from build123d import *

# Parameters (mm, degrees)
SKETCH1_W           = 30
SKETCH1_H           = 30
BOSS_EXTRUDE1_DEPTH = 2
SKETCH2_R           = 1.8
CUT_EXTRUDE1_DEPTH  = 22.307275753
FILLET1_R           = 3
CUT_EXTRUDE2_DEPTH  = 22.307275753


with BuildPart() as part:
    # Sketch1 → Boss-Extrude1 (new body)
    with BuildSketch(Plane.XY):
        Rectangle(SKETCH1_W, SKETCH1_H)
    extrude(amount=BOSS_EXTRUDE1_DEPTH)

    # Sketch2 → Cut-Extrude1 (cut, through all)
    with BuildSketch(Plane.XY.offset(2)):
        with Locations((-12, 12)):
            Circle(SKETCH2_R)
        with Locations((12, 12)):
            Circle(SKETCH2_R)
        with Locations((12, -12)):
            Circle(SKETCH2_R)
        with Locations((-12, -12)):
            Circle(SKETCH2_R)
    extrude(amount=-CUT_EXTRUDE1_DEPTH, mode=Mode.SUBTRACT)

    # Fillet1
    fillet1_edges = [part.edges().sort_by_distance(p)[0] for p in [
        (15, -15, 1),
        (-15, -15, 1),
        (-15, 15, 1),
        (15, 15, 1),
    ]]
    fillet(fillet1_edges, radius=FILLET1_R)

    # Sketch3 → Cut-Extrude2 (cut, through all)
    with BuildSketch(Plane.XY.offset(2)):
        with BuildLine():
            Line((-7.937253933, 1), (-9.949874371, 1))
            ThreePointArc((-9.949874371, 1), (-7.071067812, 7.071067812), (-1, 9.949874371))
            Line((-1, 9.949874371), (-1, 7.937253933))
            ThreePointArc((-1, 7.937253933), (-5.656854249, 5.656854249), (-7.937253933, 1))
        make_face()
        with BuildLine():
            Line((-1, -3.872983346), (-1, -5.916079783))
            ThreePointArc((-1, -5.916079783), (-4.242640687, -4.242640687), (-5.916079783, -1))
            Line((-5.916079783, -1), (-3.872983346, -1))
            ThreePointArc((-3.872983346, -1), (-2.828427125, -2.828427125), (-1, -3.872983346))
        make_face()
        with BuildLine():
            Line((-3.872983346, 1), (-5.916079783, 1))
            ThreePointArc((-5.916079783, 1), (-4.242640687, 4.242640687), (-1, 5.916079783))
            Line((-1, 5.916079783), (-1, 3.872983346))
            ThreePointArc((-1, 3.872983346), (-2.828427125, 2.828427125), (-3.872983346, 1))
        make_face()
        with BuildLine():
            Line((3.872983346, -1), (5.916079783, -1))
            ThreePointArc((5.916079783, -1), (4.242640687, -4.242640687), (1, -5.916079783))
            Line((1, -5.916079783), (1, -3.872983346))
            ThreePointArc((1, -3.872983346), (2.828427125, -2.828427125), (3.872983346, -1))
        make_face()
        with BuildLine():
            Line((3.872983346, 1), (5.916079783, 1))
            ThreePointArc((5.916079783, 1), (4.242640687, 4.242640687), (1, 5.916079783))
            Line((1, 5.916079783), (1, 3.872983346))
            ThreePointArc((1, 3.872983346), (2.828427125, 2.828427125), (3.872983346, 1))
        make_face()
        with BuildLine():
            Line((-11.958260743, 1), (-13.964240044, 1))
            ThreePointArc((-13.964240044, 1), (-9.899494937, 9.899494937), (-1, 13.964240044))
            Line((-1, 13.964240044), (-1, 11.958260743))
            ThreePointArc((-1, 11.958260743), (-8.485281374, 8.485281374), (-11.958260743, 1))
        make_face()
        with BuildLine():
            Line((1, 11.958260743), (1, 13.964240044))
            ThreePointArc((1, 13.964240044), (9.899494937, 9.899494937), (13.964240044, 1))
            Line((13.964240044, 1), (11.958260743, 1))
            ThreePointArc((11.958260743, 1), (8.485281374, 8.485281374), (1, 11.958260743))
        make_face()
        with BuildLine():
            Line((1, 7.937253933), (1, 9.949874371))
            ThreePointArc((1, 9.949874371), (7.071067812, 7.071067812), (9.949874371, 1))
            Line((9.949874371, 1), (7.937253933, 1))
            ThreePointArc((7.937253933, 1), (5.656854249, 5.656854249), (1, 7.937253933))
        make_face()
        with BuildLine():
            Line((7.937253933, -1), (9.949874371, -1))
            ThreePointArc((9.949874371, -1), (7.071067812, -7.071067812), (1, -9.949874371))
            Line((1, -9.949874371), (1, -7.937253933))
            ThreePointArc((1, -7.937253933), (5.656854249, -5.656854249), (7.937253933, -1))
        make_face()
        with BuildLine():
            Line((11.958260743, -1), (13.964240044, -1))
            ThreePointArc((13.964240044, -1), (9.899494937, -9.899494937), (1, -13.964240044))
            Line((1, -13.964240044), (1, -11.958260743))
            ThreePointArc((1, -11.958260743), (8.485281374, -8.485281374), (11.958260743, -1))
        make_face()
        with BuildLine():
            Line((-1, -11.958260743), (-1, -13.964240044))
            ThreePointArc((-1, -13.964240044), (-9.899494937, -9.899494937), (-13.964240044, -1))
            Line((-13.964240044, -1), (-11.958260743, -1))
            ThreePointArc((-11.958260743, -1), (-8.485281374, -8.485281374), (-1, -11.958260743))
        make_face()
        with BuildLine():
            Line((-1, -7.937253933), (-1, -9.949874371))
            ThreePointArc((-1, -9.949874371), (-7.071067812, -7.071067812), (-9.949874371, -1))
            Line((-9.949874371, -1), (-7.937253933, -1))
            ThreePointArc((-7.937253933, -1), (-5.656854249, -5.656854249), (-1, -7.937253933))
        make_face()
    extrude(amount=-CUT_EXTRUDE2_DEPTH, mode=Mode.SUBTRACT)


solid = part.part
Source: CAD feature listing. Evaluate the final solid. Frame: model axes, mm. A direction names the side the tool comes from. Coordinates: 2 decimals unless noted, no trailing zeros. Order: outer loops, then holes, each group sorted by start corner. A loop starts at its lowest first (then second) coordinate and runs counter-clockwise, first axis right, second up.
Item 1: Material intervals for line 1 (Y direction, x = 12.5, z = 0.15); line 2 (Y direction, x = -12, z = 0.45), sorted ascending.
Output values:
line 1: y = -14.96 to -13.73, -10.27 to -6.3, -1 to 1, 6.3 to 10.27, 13.73 to 14.96
line 2: y = -15 to -13.8, -10.2 to -7.21, -1 to 1, 7.21 to 10.2, 13.8 to 15
Item 2: Cut plane A-A (y = -2). Return loops of the section in (x, z), plus the area to 3 significant figures.
Output values:
outline: (-15, 0) - (-13.86, 0) - (-13.86, 2) - (-15, 2) - close; (-11.83, 0) - (-9.8, 0) - (-9.8, 2) - (-11.83, 2) - close; (-7.75, 0) - (-5.66, 0) - (-5.66, 2) - (-7.75, 2) - close; (-3.46, 0) - (3.46, 0) - (3.46, 2) - (-3.46, 2) - close; (5.66, 0) - (7.75, 0) - (7.75, 2) - (5.66, 2) - close; (9.8, 0) - (11.83, 0) - (11.83, 2) - (9.8, 2) - close; (13.86, 0) - (15, 0) - (15, 2) - (13.86, 2) - close
area: 34.9 mm2
Item 3: Cut plane D-D (x = -5). Return loops of the section in (y, z) (3 decimals).
Output values:
outline: (-15, 0) - (-13.077, 0) - (-13.077, 2) - (-15, 2) - close; (-10.909, 0) - (-8.66, 0) - (-8.66, 2) - (-10.909, 2) - close; (-6.245, 0) - (-3.317, 0) - (-3.317, 2) - (-6.245, 2) - close; (-1, 0) - (1, 0) - (1, 2) - (-1, 2) - close; (3.317, 0) - (6.245, 0) - (6.245, 2) - (3.317, 2) - close; (8.66, 0) - (10.909, 0) - (10.909, 2) - (8.66, 2) - close; (13.077, 0) - (15, 0) - (15, 2) - (13.077, 2) - close
Item 4: First-contact query: P1, Ø8, axis at x = 2, y = 2, coming from the -Z side; P2, Ø0.6, axis at y = -12.5, z = 0.5, coming from the +X side. Flat tips, straight axial feed; report the tip coordinate or a pass-through.
Output values:
P1: stops at z = 0
P2: stops at x = 14.99
Item 5: Set-up query: faces 1 (the face through (1, 5, 1)), 2 (the face through (0, 0, 0)). Return all of +Z, -Z, +X, -X, +Y, -Y with unobstructed straight access to the full face (end or side cutting, diameter ignored); none if empty.
Output values:
face 1: +Z, -Z
face 2: -Z, +X, -X, +Y, -Y
Item 6: Pull-direction query (Y, two-part tool) for faces 3 (the face through (15, 0, 1)), 4 (the face through (7.14, -7, 1.01)); classes: pulls with the +Y half, pulls with the -Y half, needs draft (parallel to the pull), parting line crosses it, or undercut.
Output values:
face 3: needs draft
face 4: undercut
Item 7: Cut plane B-B (x = 7). Return loops of the section in (y, z), plus the area to 3 significant figures.
Output values:
outline: (-15, 0) - (-12.12, 0) - (-12.12, 2) - (-15, 2) - close; (-9.75, 0) - (-7.14, 0) - (-7.14, 2) - (-9.75, 2) - close; (-3.87, 0) - (3.87, 0) - (3.87, 2) - (-3.87, 2) - close; (7.14, 0) - (9.75, 0) - (9.75, 2) - (7.14, 2) - close; (12.12, 0) - (15, 0) - (15, 2) - (12.12, 2) - close
area: 37.4 mm2
Item 8: Cut plane C-C (y = -11.5). Return loops of the section in (x, z), plus the area to 3 significant figures.
Output values:
outline: (-15, 0) - (-13.73, 0) - (-13.73, 2) - (-15, 2) - close; (-10.27, 0) - (-7.98, 0) - (-7.98, 2) - (-10.27, 2) - close; (-3.43, 0) - (3.43, 0) - (3.43, 2) - (-3.43, 2) - close; (7.98, 0) - (10.27, 0) - (10.27, 2) - (7.98, 2) - close; (13.73, 0) - (15, 0) - (15, 2) - (13.73, 2) - close
area: 27.9 mm2
